from build123d import *

# Parameters (mm, degrees)
SKETCH_1_W          = 60
SKETCH_1_H          = 37
SKETCH_1_R          = 1.75
EXTRUDE_1_DEPTH     = 4
SKETCH_2_W          = 20
SKETCH_2_H          = 10
SKETCH_2_H_2        = 15
EXTRUDE_2_DEPTH     = 10
SKETCH_3_W          = 20
SKETCH_3_H          = 62
EXTRUDE_3_DEPTH     = 4
SKETCH_4_W          = 6
SKETCH_4_H          = 15
EXTRUDE_4_DEPTH     = 5
CUT_EXTRUDE_1_REACH = 66.655
SKETCH_4_3_R        = 2.25
SKETCH_5_W          = 30
SKETCH_5_H          = 38
CUT_EXTRUDE_2_DEPTH = 67.221220164
EXTRUDE_7_DEPTH     = 4
FILLET_1_R          = 3


with BuildPart() as part:
    # 草图1 → 凸台-拉伸1 (new body)
    with BuildSketch(Plane(origin=(0, 0, 0), x_dir=(1, 0, 0), z_dir=(0, 1, 0))):
        Polygon((-30, 22), (-30, 40), (-47.5, 40), (-47.5, -40), (47.5, -40), (47.5, 40), (30, 40), (30, 22), align=None)
        with Locations((0, -11.5)):
            Rectangle(SKETCH_1_W, SKETCH_1_H, mode=Mode.SUBTRACT)
        with Locations(Location((-44, 36.5, 0), (0, 0, 270))):
            Circle(SKETCH_1_R, mode=Mode.SUBTRACT)
        with Locations(Location((44, 36.5, 0), (0, 0, 270))):
            Circle(SKETCH_1_R, mode=Mode.SUBTRACT)
        with Locations(Location((-44, -28.5, 0), (0, 0, 270))):
            Circle(SKETCH_1_R, mode=Mode.SUBTRACT)
        with Locations(Location((44, -28.5, 0), (0, 0, 270))):
            Circle(SKETCH_1_R, mode=Mode.SUBTRACT)
    extrude(amount=EXTRUDE_1_DEPTH)

    # 草图2 → 凸台-拉伸2 (add)
    with BuildSketch(Plane.XZ):
        with Locations((0, 35)):
            Rectangle(SKETCH_2_W, SKETCH_2_H)
        with Locations((0, -14.5)):
            Rectangle(SKETCH_2_W, SKETCH_2_H_2)
    extrude(amount=EXTRUDE_2_DEPTH)

    # 草图3 → 凸台-拉伸3 (add)
    with BuildSketch(Plane.XZ.offset(10)):
        with Locations((0, 9)):
            Rectangle(SKETCH_3_W, SKETCH_3_H)
    extrude(amount=EXTRUDE_3_DEPTH)

    # 草图4 → 凸台-拉伸4 (add)
    with BuildSketch(Plane.XZ.offset(14)):
        with Locations((0, 32.5)):
            Rectangle(SKETCH_4_W, SKETCH_4_H)
        with Locations((0, -14.5)):
            Rectangle(SKETCH_4_W, SKETCH_4_H)
    extrude(amount=EXTRUDE_4_DEPTH)

    # 草图4<3> → 切除-拉伸1 (cut, up to next)
    with BuildSketch(Plane.XZ.offset(14), mode=Mode.PRIVATE) as cut_extrude_1_sk1:
        with Locations(Location((0, 12, 0), (0, 0, 270))):
            Circle(SKETCH_4_3_R)
    cut_extrude_1_tool1 = extrude(cut_extrude_1_sk1.sketch, amount=-CUT_EXTRUDE_1_REACH, mode=Mode.PRIVATE) & part.part
    add(cut_extrude_1_tool1.solids().sort_by_distance((0, -14, 12))[0], mode=Mode.SUBTRACT)

    # 草图5 → 切除-拉伸2 (cut, through all)
    with BuildSketch(Plane(origin=(0, 4, 0), x_dir=(1, 0, 0), z_dir=(0, 1, 0))):
        with Locations((-32.5, -1)):
            Rectangle(SKETCH_5_W, SKETCH_5_H)
    extrude(amount=-CUT_EXTRUDE_2_DEPTH, mode=Mode.SUBTRACT)

    # 草图6 → 凸台-拉伸7 (add)
    with BuildSketch(Plane(origin=(0, 4, 0), x_dir=(1, 0, 0), z_dir=(0, 1, 0))):
        Polygon((-10.5, 7), (-17.5, 7), (-17.5, -20), (-30, -20), (-30, -30), (-10.5, -30), align=None)
    extrude(amount=-EXTRUDE_7_DEPTH)

    # 圆角1
    fillet_1_edges = [part.edges().sort_by_distance(p)[0] for p in [
        (-30, 2, -22),
    ]]
    fillet(fillet_1_edges, radius=FILLET_1_R)
    fillet_1_2_edges = [part.edges().sort_by_distance(p)[0] for p in [
        (-30, 2, -40),
    ]]
    fillet(fillet_1_2_edges, radius=FILLET_1_R)
    fillet_1_3_edges = [part.edges().sort_by_distance(p)[0] for p in [
        (30, 2, -7),
    ]]
    fillet(fillet_1_3_edges, radius=FILLET_1_R)
    fillet_1_4_edges = [part.edges().sort_by_distance(p)[0] for p in [
        (30, 2, 30),
    ]]
    fillet(fillet_1_4_edges, radius=FILLET_1_R)
    fillet_1_5_edges = [part.edges().sort_by_distance(p)[0] for p in [
        (-10.5, 2, 30),
    ]]
    fillet(fillet_1_5_edges, radius=FILLET_1_R)
    fillet_1_6_edges = [part.edges().sort_by_distance(p)[0] for p in [
        (30, 2, -40),
    ]]
    fillet(fillet_1_6_edges, radius=FILLET_1_R)
    fillet_1_7_edges = [part.edges().sort_by_distance(p)[0] for p in [
        (30, 2, -22),
    ]]
    fillet(fillet_1_7_edges, radius=FILLET_1_R)
    fillet_1_8_edges = [part.edges().sort_by_distance(p)[0] for p in [
        (47.5, 2, -40),
    ]]
    fillet(fillet_1_8_edges, radius=FILLET_1_R)
    fillet_1_9_edges = [part.edges().sort_by_distance(p)[0] for p in [
        (47.5, 2, 40),
    ]]
    fillet(fillet_1_9_edges, radius=FILLET_1_R)
    fillet_1_10_edges = [part.edges().sort_by_distance(p)[0] for p in [
        (-47.5, 2, 40),
    ]]
    fillet(fillet_1_10_edges, radius=FILLET_1_R)
    fillet_1_11_edges = [part.edges().sort_by_distance(p)[0] for p in [
        (-47.5, 2, 20),
    ]]
    fillet(fillet_1_11_edges, radius=FILLET_1_R)
    fillet_1_12_edges = [part.edges().sort_by_distance(p)[0] for p in [
        (-17.5, 2, 20),
    ]]
    fillet(fillet_1_12_edges, radius=FILLET_1_R)
    fillet_1_13_edges = [part.edges().sort_by_distance(p)[0] for p in [
        (-17.5, 2, -18),
    ]]
    fillet(fillet_1_13_edges, radius=FILLET_1_R)
    fillet_1_14_edges = [part.edges().sort_by_distance(p)[0] for p in [
        (-47.5, 2, -18),
    ]]
    fillet(fillet_1_14_edges, radius=FILLET_1_R)
    fillet_1_15_edges = [part.edges().sort_by_distance(p)[0] for p in [
        (-47.5, 2, -40),
    ]]
    fillet(fillet_1_15_edges, radius=FILLET_1_R)
    fillet_1_16_edges = [part.edges().sort_by_distance(p)[0] for p in [
        (-10.5, 2, -7),
    ]]
    fillet(fillet_1_16_edges, radius=FILLET_1_R)


solid = part.part
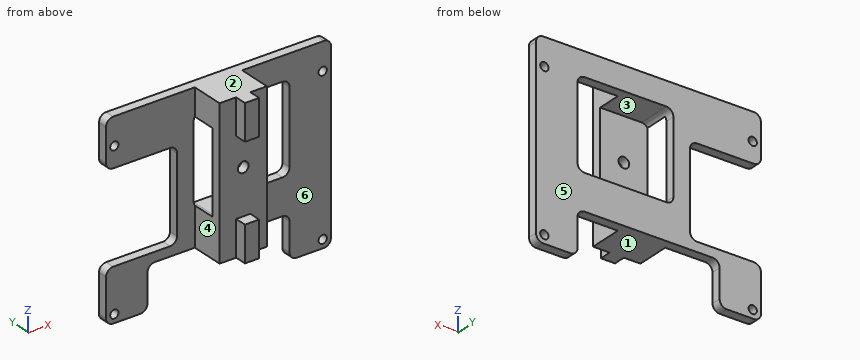
Geometry: final body of the model. Coordinates: model frame, mm. Face numbers are marked on the shaded views. A direction names the side the tool comes from. Round coordinates to 2 decimals unless told otherwise and drop trailing zeros. Order: outer loops, then holes, each group sorted by start corner. A loop starts at its lowest first (then second) coordinate and runs counter-clockwise, first axis right, second up.
Q1. Pin query (flat end, axial travel): pin 1 (4 mm diameter, centred on x = -5.5, y = -2, fed in from -Z); pin 2 (1.2 mm diameter, centred on y = 1.5, z = 17, fed in from -X); pin 3 (5 mm diameter, centred on y = -3.5, z = 10, fed in from -X); pin 4 (1.5 mm diameter, centred on y = -16.5, z = 31, fed in from +X). Return the tip coordinate at first contact, or that it passes through.
Result sheet:
pin 1: stops at z = -22
pin 2: stops at x = -17.56
pin 3: passes through
pin 4: stops at x = 3
Q2. Access query for the marked faces 4, 5 and 6. Directions: +Z, -Z, +X, -X, +Y, -Y. A direction counts if a zero-diameter tool reaches every point of the face in a straight line with its end or side. Return the directions, or none.
Result sheet:
face 4: +Z, -Z, -X, -Y
face 5: +Z, -Z, +X, -X, +Y
face 6: +Z, -Z, +X, -Y
Q3. Mould query, pull axis Z, two halves, no side actions, for the marked faces 1, 2 and 3. Classes: released by +Z, released by -Z, zero draft, split by the parting line, or undercut.
Result sheet:
face 1: released by -Z
face 2: released by +Z
face 3: undercut
Q4. Section B-B, the plane z = -26.5. Output: boundary loops of the cut face in (x, y).
Result sheet:
outline: (-47.5, 0) - (-30, 0) - (-30, 4) - (-47.5, 4) - close; (30, 0) - (47.5, 0) - (47.5, 4) - (30, 4) - close
Q5. Material intervals for probe 1 along Z at (x, y) = (-25.5, 0.5); probe 2 along X at (y, z) = (2.9, 28.5); probe 3 along X at (y, z) = (-3.5, 35.5), sorted ascending.
Result sheet:
probe 1: z = -22 to -18, 20 to 40
probe 2: x = -47.5 to -45.75, -42.25 to -10.1, 29.6 to 42.25, 45.75 to 47.5
probe 3: x = -10 to 10
Q6. Section A-A, the plane x = -37.5. Output: boundary loops of the cut face in (y, z).
Result sheet:
outline: (0, -40) - (4, -40) - (4, -18) - (0, -18) - close; (0, 20) - (4, 20) - (4, 40) - (0, 40) - close
Q7. Section D-D, the plane y = -12.5. Output: boundary loops of the cut face in (x, z), and give its area (3 significant figures).
Result sheet:
outline: (-10, -22) - (10, -22) - (10, 40) - (-10, 40) - close; hole circle Ø4.5 at (0, 12)
area: 1,220 mm2
Q8. Section C-C, the plane z = 12. Output: boundary loops of the cut face in (x, y), and give its area (3 significant figures).
Result sheet:
outline: (-17.5, 0) - (-10.5, 0) - (-10.5, 4) - (-17.5, 4) - close; (-10, -14) - (-2.25, -14) - (-2.25, -10) - (-10, -10) - close; (2.25, -14) - (10, -14) - (10, -10) - (2.25, -10) - close; (30, 0) - (47.5, 0) - (47.5, 4) - (30, 4) - close
area: 160 mm2
